Check sheet for the drawn part. Datum: minimum x, y, z corner. Units: mm. Give positions to 0.01 mm unless a question says otherwise; leave off trailing zeros. Order: outer loops, then holes, each group sorted by start corner. A loop starts at its lowest first (then second) coordinate and runs counter-clockwise, first axis right, second up.
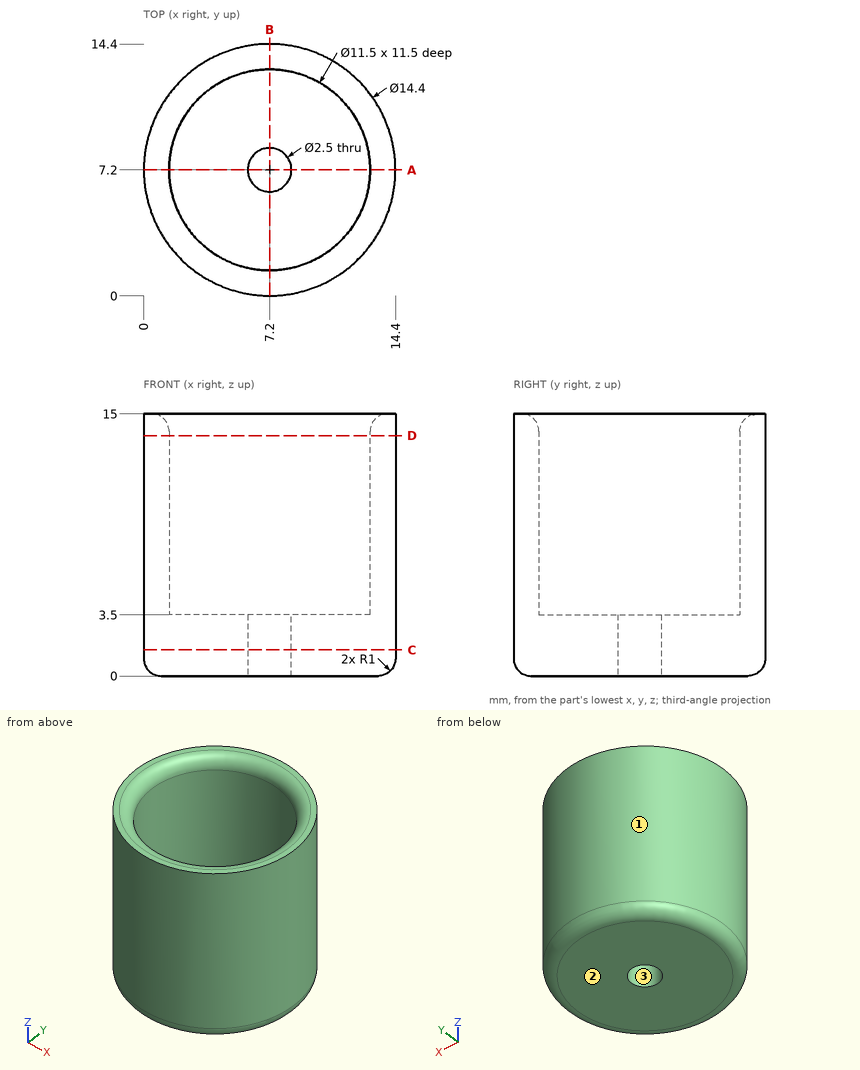
Item 1: Sectioned sample at A-A (y = 7.2). Enter the section's corners in (x, z), and give its area (3 significant figures).
Reported:
outline: (0, 1) arc R1 ccw to (1, 0) - (5.95, 0) - (5.95, 3.5) - (1.45, 3.5) - (1.45, 14) arc R1 ccw to (0.45, 15) - (0, 15) - close; (8.45, 0) - (13.4, 0) arc R1 ccw to (14.4, 1) - (14.4, 15) - (13.95, 15) arc R1 ccw to (12.95, 14) - (12.95, 3.5) - (8.45, 3.5) - close
area: 74.1 mm2
Item 2: Scan lines: L1, parallel to Y at x = 7.2, z = 1.05; L2, parallel to Y at x = 7.2, z = 8.5; L3, parallel to Z at x = 11.5, y = 7.75. Record each from-to range of solid material in increasing order.
Reported:
L1: y = 0 to 5.95, 8.45 to 14.4
L2: y = 0 to 1.45, 12.95 to 14.4
L3: z = 0 to 3.5
Item 3: Sectioned sample at D-D (z = 13.75). Enter the section's corners in (x, y).
Reported:
outline: circle Ø14.4 at (7.2, 7.2); hole circle Ø11.5 at (7.2, 7.2)
Item 4: Gauge pin test, flat ends, axial feed: pin 1 (6 mm diameter, centred on x = 8, y = 5, fed in from +Z); pin 2 (6 mm diameter, centred on y = 12.5, z = 11.5, fed in from +X); pin 3 (8 mm diameter, centred on y = 2, z = 7.5, fed in from -X). Record the tip position at first contact, or that the pin passes through.
Reported:
pin 1: stops at z = 3.5
pin 2: stops at x = 14.02
pin 3: stops at x = 0.1
Item 5: Draft check along X on the marked faces 1, 2 and 3. Enter one of: released by +X, released by -X, zero draft, split by the parting line, or undercut.
Reported:
face 1: split by the parting line
face 2: zero draft
face 3: undercut
Item 6: Sectioned sample at C-C (z = 1.5). Enter the section's corners in (x, y).
Reported:
outline: circle Ø14.4 at (7.2, 7.2); hole circle Ø2.5 at (7.2, 7.2)
